Read the model definition and answer for the solid it produces. Units are mm, in the model's axes. Give positions to 0.01 mm unless a question says otherwise; leave off trailing zeros. Write each loop counter-clockwise with the first axis right and the second up, starting at its lowest first coordinate (ties: lowest second). Pieces come first, ordered by that corner, then holes. Notation, with made-up numbers: M 43,44.5 L 57,44.5 A30 cw 57,69.5 Z; hole C 10,-20.5 d4. An arc over 180 degrees is marked long. Put each result on its own line as item: value.
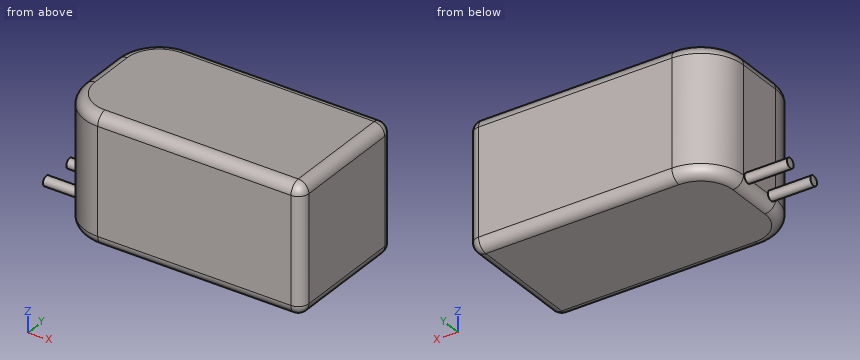
from build123d import *

# Parameters (mm, degrees)
SKETCH1_W           = 58
SKETCH1_H           = 30
BOSS_EXTRUDE1_DEPTH = 31
FILLET1_R           = 10
FILLET2_R           = 2.5
SKETCH2_R           = 1.15
BOSS_EXTRUDE2_DEPTH = 10


with BuildPart() as part:
    # Sketch1 → Boss-Extrude1 (new body)
    with BuildSketch(Plane(origin=(0, 0, 0), x_dir=(1, 0, 0), z_dir=(0, 1, 0))):
        Rectangle(SKETCH1_W, SKETCH1_H)
    extrude(amount=BOSS_EXTRUDE1_DEPTH)

    # Fillet1
    fillet1_edges = [part.edges().sort_by_distance(p)[0] for p in [
        (-29, 31, 0),
        (-29, 0, 0),
    ]]
    fillet(fillet1_edges, radius=FILLET1_R)

    # Fillet2
    fillet2_edges = [part.edges().sort_by_distance(p)[0] for p in [
        (-29, 15.5, 15),
        (-29, 15.5, -15),
        (5, 0, 15),
        (5, 31, 15),
        (-26.071067812, 28.071067812, 15),
        (-26.071067812, 2.928932188, 15),
        (-26.071067812, 28.071067812, -15),
        (-26.071067812, 2.928932188, -15),
        (29, 31, 0),
        (5, 0, -15),
        (29, 0, 0),
        (5, 31, -15),
        (29, 15.5, 15),
        (29, 15.5, -15),
    ]]
    fillet(fillet2_edges, radius=FILLET2_R)

    # Sketch2 → Boss-Extrude2 (add)
    with BuildSketch(Plane.ZY.offset(29)):
        with Locations((-12.5, 19.5)):
            Circle(SKETCH2_R)
        with Locations((-12.5, 11.5)):
            Circle(SKETCH2_R)
    extrude(amount=BOSS_EXTRUDE2_DEPTH)


solid = part.part
(1) Section B-B on y = 19.5 is taken. Determine the outline of the cut face in (x, z).
Result:
outline: M -39,-13.65 L -29,-13.65 L -29,-12.5 A2.5 ccw -26.5,-15 L 26.5,-15 A2.5 ccw 29,-12.5 L 29,12.5 A2.5 ccw 26.5,15 L -26.5,15 A2.5 ccw -29,12.5 L -29,-11.35 L -39,-11.35 Z
(2) Section C-C on x = -34.5 is taken. Determine the outline of the cut face in (y, z).
Result:
outline: C 11.5,-12.5 d2.3; C 19.5,-12.5 d2.3
(3) Given pin 1 Ø5 at (y, z) = (16.5, 10.5) entering from -X; pin 2 Ø0.9 at (y, z) = (19, -13) entering from +X; pin 3 Ø1 at (y, z) = (23.5, -2) entering from -X, each flat-ended and moving along its own axis, determine where each tip first touches the part or whether it passes through.
Result:
pin 1: stops at x = -29
pin 2: stops at x = 29
pin 3: stops at x = -28.8
(4) Straight lines are drawn through the part: line 1 along X through (y, z) = (10, -11.25); line 2 along Z through (x, y) = (-30, 19.5); line 3 along Y through (x, z) = (-0.5, 13.75). For each, find the intervals that lie inside material, in ascending order. Write a range as from..to.
Result:
line 1: x = -29..29
line 2: z = -13.65..-11.35
line 3: y = 0.33..30.67
(5) Section A-A on z = 1 is taken. Determine the outline of the cut face in (x, y).
Result:
outline: M -29,10 A10 ccw -19,0 L 26.5,0 A2.5 ccw 29,2.5 L 29,28.5 A2.5 ccw 26.5,31 L -19,31 A10 ccw -29,21 Z
(6) Section D-D on y = 14 is taken. Determine the outline of the cut face in (x, z).
Result:
outline: M -29,-12.5 A2.5 ccw -26.5,-15 L 26.5,-15 A2.5 ccw 29,-12.5 L 29,12.5 A2.5 ccw 26.5,15 L -26.5,15 A2.5 ccw -29,12.5 Z
